Autodesk Inventor part; units mm, degrees
ref_plane "YZ Plane" through (0, 0, 0) normal (1, 0, 0) x (0, 1, 0)
ref_plane "XZ Plane" through (0, 0, 0) normal (0, 1, 0) x (-1, 0, 0)
ref_plane "XY Plane" through (0, 0, 0) normal (0, 0, 1) x (1, 0, 0)
sketch "Sketch1" plane through (0, 0, 0) normal (0, 0, 1) x (1, 0, 0)
  line L0 (-216.6526, -262.3711) -> (123.3474, -262.3711)
  line L1 (123.3474, -262.3711) -> (123.3474, 7.6289)
  line L2 (123.3474, 7.6289) -> (-216.6526, 7.6289)
  line L3 (-216.6526, 7.6289) -> (-216.6526, -262.3711)
  point P0 (0, 0)
  dimension "d0" = 340
  dimension "d1" = 270
extrude "Extrusion1" add sketch "Sketch1" along normal blind 10
sketch "Sketch2" plane through (0, 0, 0) normal (0, 0, -1) x (-1, 0, 0)
  line L0 (-66.3474, -50.3711) -> (-66.3474, -52.3711) construction
  line L1 (-66.3474, -52.3711) -> (-47.3474, -52.3711) construction
  line L2 (-47.3474, -52.3711) -> (-47.3474, -37.3711) construction
  line L3 (-47.3474, -37.3711) -> (-64.7974, -37.3711) construction
  line L4 (-64.7974, -37.3711) -> (-64.7974, -42.3711) construction
  line L5 (-64.7974, -42.3711) -> (-79.8974, -42.3711) construction
  line L6 (-79.8974, -42.3711) -> (-79.8974, -37.3711) construction
  line L7 (-79.8974, -37.3711) -> (-97.3474, -37.3711) construction
  line L8 (-97.3474, -37.3711) -> (-97.3474, -52.3711) construction
  line L9 (-97.3474, -52.3711) -> (-78.3474, -52.3711) construction
  line L10 (-78.3474, -52.3711) -> (-78.3474, -50.3711) construction
  line L11 (-78.3474, -50.3711) -> (-66.3474, -50.3711) construction
  line L12 (-79.7974, -42.3711) -> (-79.7974, -9.1428) construction
  line L13 (-64.7974, -42.3711) -> (-79.7974, -42.3711) construction
  line L14 (-64.7974, -42.3711) -> (-64.7974, -9.1428) construction
  line L15 (-79.7974, -26.2239) -> (-79.7974, -29.3711) construction
  line L16 (-79.7974, -29.3711) -> (-64.7974, -29.3711) construction
  line L17 (-64.7974, -29.3711) -> (-64.7974, -26.2239) construction
  line L18 (-64.7974, -26.2239) -> (-79.7974, -26.2239) construction
  line L19 (-79.7974, 7.2343) -> (-64.7974, 7.2343) construction
  line L20 (-79.7974, -9.1428) -> (-79.7974, 7.2343) construction
  line L21 (-64.7974, 7.2343) -> (-64.7974, -9.1428) construction
  line L22 (-123.3474, 7.6289) -> (216.6526, 7.6289)
  line L23 (-79.9974, 7.6289) -> (-79.9974, -37.1711)
  line L24 (-79.9974, -37.1711) -> (-97.5474, -37.1711)
  line L25 (-97.5474, -37.1711) -> (-97.5474, -52.5711)
  line L26 (-97.5474, -52.5711) -> (-47.1474, -52.5711)
  line L27 (-47.1474, -52.5711) -> (-47.1474, -37.1711)
  line L28 (-47.1474, -37.1711) -> (-64.5974, -37.1711)
  line L29 (-64.5974, -37.1711) -> (-64.5974, 7.6289)
  line L30 (-79.9974, 7.6289) -> (-64.5974, 7.6289)
  circle A0 centre (-57.3474, -44.8711) radius 1.621
  circle A1 centre (-87.3474, -44.8711) radius 1.621
  line L31 (-64.7974, -9.1428) -> (-79.7974, -9.1428)
  line L32 (-64.7974, -9.1428) -> (-79.7974, -9.1428)
  circle A2 centre (-72.2869, -16.8711) radius 1.621
  circle A3 centre (-72.2869, -36.8711) radius 1.621
  point P0 (0, 0)
  dimension "d4" = 0.2
  dimension "d5" = 0.2
  dimension "d6" = 0.2
  dimension "d7" = 0.2
  dimension "d8" = 0.2
  dimension "d9" = 0.2
extrude "Extrusion2" cut sketch "Sketch2" against normal blind 5 contours L22 L29 L28 L27 L26 L25 L24 L23 | A0 | A1 | A2 | A3
sketch "Sketch4" plane through (0, 0, 0) normal (0, 0, -1) x (-1, 0, 0)
  circle A0 centre (-48.2081, -38.2317) radius 2
  line L0 (-47.1474, -37.1711) -> (-47.1474, -52.5711)
  line L1 (-47.1474, -37.1711) -> (-48.0356, -38.0592) construction
  line L2 (-64.5974, -37.1711) -> (-47.1474, -37.1711)
  circle A1 centre (-48.2081, -51.5104) radius 2
  circle A2 centre (-96.4868, -51.5104) radius 2
  circle A3 centre (-96.4868, -38.2317) radius 2
  line L3 (-47.1474, -52.5711) -> (-49.4974, -50.2211) construction
  line L4 (-47.1474, -52.5711) -> (-97.5474, -52.5711)
  line L5 (-97.5474, -52.5711) -> (-95.2238, -50.2474) construction
  line L6 (-97.5474, -37.1711) -> (-95.2759, -39.4427) construction
  line L7 (-97.5474, -52.5711) -> (-97.5474, -37.1711)
  point P0 (0, 0)
  dimension "d17" = 4
  dimension "d18" = 45
  dimension "d19" = 1.5
  dimension "d20" = 4
  dimension "d21" = 4
  dimension "d22" = 4
  dimension "d23" = 45
  dimension "d24" = 45
  dimension "d25" = 1.5
  dimension "d26" = 1.5
  dimension "d27" = 1.5
extrude "Extrusion4" cut sketch "Sketch4" against normal up to surface (5 mm away)
equation "\"d20\" = d17"
equation "\"d21\" = d17"
equation "\"d22\" = d17"
equation "\"d25\" = d19"
equation "\"d26\" = d19"
equation "\"d27\" = d19"
properties part number "baseplate" material "Aluminum 6061-AHC"
Geometry: final body of the model. Coordinates: model frame, mm. Round coordinates to 2 decimals unless told otherwise and drop trailing zeros. Order: outer loops, then holes, each group sorted by start corner. A loop starts at its lowest first (then second) coordinate and runs counter-clockwise, first axis right, second up. Notation, with made-up numbers: (83, 14) -> (97, 14) arc R22 cw to (97, 29) -> close; hole circle Ø5 at (4.25, 55.25). An arc over 180 degrees is marked (long way). Put each result on its own line as item: value. Start each with the question number.
Q1. Line query: probe 1 along X at (y, z) = (-31.5, 3). Output: solid intervals per line, ascending.
Q2. First-contact query: pin 1 (6.5 mm diameter, centred on x = 48.21, y = -38.23, fed in from -Z); pin 2 (2.5 mm diameter, centred on x = 48.21, y = -51.51, fed in from -Z). Flat tips, straight axial feed; report the tip coordinate or a pass-through.
Q3. Section A-A on y = -23.5. Return the cut outline in (x, z).
Q4. Pull-direction query (Y, two-part tool) for faces 1 (the flat face through (-44, 7.629, 5)), 2 (the flat face through (73, -29, 5)), 3 (the flat face through (-49, -262.371, 5)), 4 (the flat face through (123.347, -129, 5)); classes: +Y half, -Y half, draft (parallel to the pull), parting line (faces both ways), or undercut.
Q5. Section C-C on z = 3.5. Return the cut outline in (x, y).
Q6. Section B-B on x = 59. Return the cut outline in (y, z).
Ans:
1. probe 1: x = -216.65 to 64.6, 80 to 123.35
2. pin 1: stops at z = 0
2. pin 2: stops at z = 5
3. outline: (-216.65, 0) -> (64.6, 0) -> (64.6, 5) -> (80, 5) -> (80, 0) -> (123.35, 0) -> (123.35, 10) -> (-216.65, 10) -> close
4. face 1: +Y half
4. face 2: undercut
4. face 3: -Y half
4. face 4: draft
5. outline: (-216.65, -262.37) -> (123.35, -262.37) -> (123.35, 7.63) -> (80, 7.63) -> (80, -37.17) -> (94.79, -37.17) arc R2 cw (long way) to (97.55, -39.93) -> (97.55, -49.81) arc R2 cw (long way) to (94.79, -52.57) -> (49.9, -52.57) arc R2 cw (long way) to (47.15, -49.81) -> (47.15, -39.93) arc R2 cw (long way) to (49.9, -37.17) -> (64.6, -37.17) -> (64.6, 7.63) -> (-216.65, 7.63) -> close
6. outline: (-262.37, 0) -> (-52.57, 0) -> (-52.57, 5) -> (-37.17, 5) -> (-37.17, 0) -> (7.63, 0) -> (7.63, 10) -> (-262.37, 10) -> close
